Verification items for the finished model (mm, model axes). A direction names the side the tool comes from. Coordinates: 2 decimals unless noted, no trailing zeros. Write each loop counter-clockwise with the first axis right and the second up, starting at its lowest first coordinate (ties: lowest second). Pieces come first, ordered by that corner, then holes. Notation, with made-up numbers: (-2.75, 71) -> (11.25, 71) arc R21 ccw to (11.25, 82) -> close; hole circle Ø11 at (-35.75, -36.5). An arc over 180 degrees is marked (long way). Answer in a Markdown table with one row per item.
```python
from build123d import *

# Parameters (mm, degrees)
SKETCH1_W            = 31.75
SKETCH1_H            = 15.875
BOSS_EXTRUDE1_DEPTH  = 4.2291
SKETCH2_W            = 29.21
SKETCH2_H            = 13.335
SKETCH2_R            = 3.175
SKETCH2_R_2          = 2.413
CUT_EXTRUDE1_DEPTH   = 7.1882
SKETCH3_R            = 2.69875
BOSS_EXTRUDE2_DEPTH  = 1.397
LPATTERN1_COUNT      = 4
LPATTERN1_PITCH      = 7.9375
LPATTERN1_COUNT_DIR2 = 2
LPATTERN1_PITCH_DIR2 = 7.9375
SKETCH2_3_R          = 3.175
SKETCH2_3_R_2        = 2.413
BOSS_EXTRUDE3_DEPTH  = 7.1882
LPATTERN2_COUNT      = 2
LPATTERN2_PITCH      = 7.9375
LPATTERN2_COL_COUNT  = 2
LPATTERN2_COL_PITCH  = 7.9375


with BuildPart() as part:
    # Sketch1 → Boss-Extrude1 (new, symmetric)
    with BuildSketch(Plane(origin=(0, 0, 0), x_dir=(1, 0, 0), z_dir=(0, 1, 0))):
        Rectangle(SKETCH1_W, SKETCH1_H)
    extrude(amount=BOSS_EXTRUDE1_DEPTH, both=True)

    # Sketch2 → Cut-Extrude1 (cut)
    with BuildSketch(Plane.XZ.offset(4.2291)):
        Rectangle(SKETCH2_W, SKETCH2_H)
        Circle(SKETCH2_R, mode=Mode.SUBTRACT)
        Circle(SKETCH2_R)
        Circle(SKETCH2_R_2, mode=Mode.SUBTRACT)
        Circle(SKETCH2_R_2)
    extrude(amount=-CUT_EXTRUDE1_DEPTH, mode=Mode.SUBTRACT)

    # Sketch3 → Boss-Extrude2 (add)
    with BuildSketch(Plane(origin=(0, 4.2291, 0), x_dir=(1, 0, 0), z_dir=(0, 1, 0))):
        with Locations(Location((11.90625, -3.96875, 0), (0, 0, 270))):
            Circle(SKETCH3_R)
    boss_extrude2 = extrude(amount=BOSS_EXTRUDE2_DEPTH)

    # LPattern1: Boss-Extrude2 4 × 2
    with Locations(*[(-i * LPATTERN1_PITCH, 0, -j * LPATTERN1_PITCH_DIR2) for i in range(LPATTERN1_COUNT) for j in range(LPATTERN1_COUNT_DIR2) if (i, j) != (0, 0)]):
        add(boss_extrude2)

    # Sketch2<3> → Boss-Extrude3 (add)
    with BuildSketch(Plane.XZ.offset(4.2291)):
        with Locations(Location((0, 0, 0), (0, 0, 270))):
            Circle(SKETCH2_3_R)
        with Locations(Location((0, 0, 0), (0, 0, 270))):
            Circle(SKETCH2_3_R_2, mode=Mode.SUBTRACT)
    boss_extrude3 = extrude(amount=-BOSS_EXTRUDE3_DEPTH)

    # LPattern2: Boss-Extrude3 ×2
    with Locations(*[(i * LPATTERN2_PITCH, 0, 0) for i in range(1, LPATTERN2_COUNT)]):
        add(boss_extrude3)

    # LPattern2 col: Boss-Extrude3 ×2
    with Locations(*[(-i * LPATTERN2_COL_PITCH, 0, 0) for i in range(1, LPATTERN2_COL_COUNT)]):
        add(boss_extrude3)


solid = part.part
```
1. Access from +Z, -Z, +X, -X, +Y, -Y to the whole of each face (thin tool, end or side, straight path). Record for faces 1 (the face through (14.582, 4.918, -4.32)), 2 (the face through (0, -1, -6.668)), 3 (the face through (-12, 5.626, 4)).
Findings below:
| item | result |
|---|---|
| face 1 | +Y |
| face 2 | -Y |
| face 3 | +Z, -Z, +X, -X, +Y |
2. Release check for a two-part mould opening along X. For faces 4 (the face through (-10.75, -0.69, -1.47)), 5 (the face through (-15.875, 0, 0)), 6 (the face through (0, 0, 7.938)) record: released by +X, released by -X, zero draft, split by the parting line, or undercut.
Findings below:
| item | result |
|---|---|
| face 4 | undercut |
| face 5 | released by -X |
| face 6 | zero draft |
3. Sectioned sample at C-C, the plane y = 5.25. Record the cut outline in (x, z), and give its area (3 significant figures).
Findings below:
| item | result |
|---|---|
| outline | circle Ø5.4 at (-11.91, -3.97); circle Ø5.4 at (-11.91, 3.97); circle Ø5.4 at (-3.97, -3.97); circle Ø5.4 at (-3.97, 3.97); circle Ø5.4 at (3.97, -3.97); circle Ø5.4 at (3.97, 3.97); circle Ø5.4 at (11.91, -3.97); circle Ø5.4 at (11.91, 3.97) |
| area | 183 mm² |
4. Sectioned sample at D-D, the plane z = -4.25. Record the cut outline in (x, y) (3 decimals), and give its area (3 significant figures).
Findings below:
| item | result |
|---|---|
| outline | (-15.875, -4.229) -> (-14.605, -4.229) -> (-14.605, 2.959) -> (14.605, 2.959) -> (14.605, -4.229) -> (15.875, -4.229) -> (15.875, 4.229) -> (14.59, 4.229) -> (14.59, 5.626) -> (9.222, 5.626) -> (9.222, 4.229) -> (6.653, 4.229) -> (6.653, 5.626) -> (1.285, 5.626) -> (1.285, 4.229) -> (-1.285, 4.229) -> (-1.285, 5.626) -> (-6.653, 5.626) -> (-6.653, 4.229) -> (-9.222, 4.229) -> (-9.222, 5.626) -> (-14.59, 5.626) -> (-14.59, 4.229) -> (-15.875, 4.229) -> close |
| area | 88.6 mm² |
5. Sectioned sample at B-B, the plane x = 0. Record the cut outline in (y, z) (1 decimal).
Findings below:
| item | result |
|---|---|
| outline | (-4.2, -7.9) -> (4.2, -7.9) -> (4.2, 7.9) -> (-4.2, 7.9) -> (-4.2, 6.7) -> (3, 6.7) -> (3, 3.2) -> (-4.2, 3.2) -> (-4.2, 2.4) -> (3, 2.4) -> (3, -2.4) -> (-4.2, -2.4) -> (-4.2, -3.2) -> (3, -3.2) -> (3, -6.7) -> (-4.2, -6.7) -> close |
6. Sectioned sample at A-A, the plane y = -3.5. Count the separate pieces of the cut face and the enclosed holes in it, and give its area (3 significant figures).
Findings below:
| item | result |
|---|---|
| separate pieces | 4 |
| enclosed holes | 4 |
| area | 155 mm² |
7. Material ranges on probe 1 along Z at (x, y) = (-7.5, 0.75); probe 2 along Z at (x, y) = (10.5, 2); probe 3 along Z at (x, y) = (11.5, -1.75), recorded low to high. Write a range as from..to.
Findings below:
| item | result |
|---|---|
| probe 1 | z = -7.94..-6.67, -3.14..-2.37, 2.37..3.14, 6.67..7.94 |
| probe 2 | z = -7.94..-6.67, -1.87..1.87, 6.67..7.94 |
| probe 3 | z = -7.94..-6.67, 6.67..7.94 |
8. Go/stop test with a flat-tipped pin: pin 1 (3 mm diameter, centred on x = 0, z = 0, fed in from -Y). Record where the tip stops, or that it passes through.
Findings below:
| item | result |
|---|---|
| pin 1 | stops at y = 2.96 |
